CAD build for the part. Positions are in the model's coordinates, mm. A direction names the side the tool comes from. Coordinates: 2 decimals unless noted, no trailing zeros. Loops run counter-clockwise (first coordinate to the right, second up) from the corner with the lowest first, then second, coordinate; pieces in that order, holes last. Notation, with made-up numbers: (30, -39.5) -> (45, -39.5) arc R33 cw to (45, -7.5) -> close; hole circle Ø1 at (5.25, -13.75). An arc over 180 degrees is marked (long way). Answer as CSV lines item,"result". Start each with the question number.
```python
from build123d import *

# Parameters (mm, degrees)
F0_R     = 1.75
F1_DEPTH = 1.6
F2_DEPTH = 7.6
F3_DEPTH = 7.5
F4_START = 2.5
F4_DEPTH = 4


with BuildPart() as f1:
    # F0 (on Front) → F1 (new body)
    with BuildSketch(Plane.XZ):
        Polygon((19.785, -8), (19.785, 8), (13.385, 8), (13.385, 1.4), (0.585, 1.4), (0.585, 8), (-19.785, 8), (-19.785, -8), align=None)
        with BuildLine():
            ThreePointArc((-15.685, 4.5846688069), (-19.135, 5), (-15.685, 5.4153311931))
            Line((-15.685, 5.4153311931), (-15.685, 6.3))
            Line((-15.685, 6.3), (-8.285, 6.3))
            Line((-8.285, 6.3), (-8.285, -6.3))
            Line((-8.285, -6.3), (-15.685, -6.3))
            Line((-15.685, -6.3), (-15.685, -5.4153311931))
            ThreePointArc((-15.685, -5.4153311931), (-19.135, -5), (-15.685, -4.5846688069))
            Line((-15.685, -4.5846688069), (-15.685, 4.5846688069))
        make_face(mode=Mode.SUBTRACT)
        with Locations((-2.515, 5)):
            Circle(F0_R, mode=Mode.SUBTRACT)
        with Locations((16.485, 5)):
            Circle(F0_R, mode=Mode.SUBTRACT)
    extrude(amount=F1_DEPTH)

    # F0 (on Front) → F2 (join)
    with BuildSketch(Plane.XZ):
        Polygon((13.385, 1.4), (13.385, 8), (1.585, 8), (1.2352894992, 8), (0.585, 8), (0.585, 1.4), align=None)
    extrude(amount=F2_DEPTH)

    # F0 (on Front) → F3 (join)
    with BuildSketch(Plane.XZ):
        with BuildLine():
            ThreePointArc((-15.685, 5.4153311931), (-15.6475449646, 5.2091650066), (-15.635, 5))
            ThreePointArc((-15.635, 5), (-15.6475449646, 4.7908349934), (-15.685, 4.5846688069))
            Line((-15.685, 4.5846688069), (-15.685, -4.5846688069))
            ThreePointArc((-15.685, -4.5846688069), (-15.6475449646, -4.7908349934), (-15.635, -5))
            ThreePointArc((-15.635, -5), (-15.6475449646, -5.2091650066), (-15.685, -5.4153311931))
            Line((-15.685, -5.4153311931), (-15.685, -6.3))
            Line((-15.685, -6.3), (-8.285, -6.3))
            Line((-8.285, -6.3), (-8.285, 6.3))
            Line((-8.285, 6.3), (-15.685, 6.3))
            Line((-15.685, 6.3), (-15.685, 5.4153311931))
        make_face()
    extrude(amount=F3_DEPTH)

    # F0 (on Front) → F4 (join)
    with BuildSketch(Plane.XZ.offset(F4_START)):
        Polygon((1.2352894992, 8), (1.585, 8), (13.585, 13), (16.585, 13), (16.585, 13.1444329156), (13.5819284966, 13.1444329156), align=None)
    extrude(amount=F4_DEPTH)


solid = f1.part
```
Q1. Probe probe 1 along X at (y, z) = (-3.5, 1.75) (3 decimals); probe 2 along Y at (x, z) = (-13, -4); probe 3 along Z at (x, y) = (15, -0.25). List the from-to ranges inside material, lowest first. Write a range as from..to.
Q2. Saw through at C-C (x = 3). List the corners of the cut face in (y, z).
Q3. Two-plate mould, pull along Z, no slides. Class faces 1 (the flat face through (-12, -7.5, 0)), 2 (the cylindrical face through (-2.89, -0.79, 3.29)), 3 (the flat face through (0, -1, -8)): pulls with the +Z half, pulls with the -Z half, needs draft (parallel to the pull), parting line crosses it, or undercut.
Q4. Saw through at D-D (z = -1.75). List the corners of the cut face in (x, y) (3 decimals).
Q5. Which spindle directions (+Z, -Z, +X, -X, +Y, -Y) get a long thin tool onto all of the face, cutting with end or side? Do faces 4 (the flat face through (-15.685, -5, 6)), 5 (the flat face through (7, -7.6, 5)), 6 (the flat face through (13.385, -5, 5)), 7 (the flat face through (-12, -5, 6.3)), 8 (the flat face through (0.585, -5, 5)). Say none if no direction does.
Q6. Saw through at B-B (x = -13). List the corners of the cut face in (y, z), and give its area (3 significant figures).
Q7. Saw through at A-A (y = -3.25). List the corners of the cut face in (x, z) (3 decimals).
Q8. Pin check, flat tips, straight feed: pin 1 Ø3 at (x, y) = (-13.5, -5.5) entering from +Z; pin 2 Ø1.8 at (y, z) = (-5.5, -1.5) entering from +X (3 decimals); pin 3 Ø1.8 at (y, z) = (-4, -2) entering from -X (3 decimals); pin 4 Ø1.5 at (x, z) = (7, 2) entering from +Y. Stop position of each tip, or through.
Ans:
1,probe 1,"x = -15.685..-8.285, 0.585..13.385"
1,probe 2,"y = -7.5..0"
1,probe 3,"z = -8..4.07, 5.93..8"
2,outline,"(-7.6, 1.4) -> (-1.6, 1.4) -> (-1.6, -8) -> (0, -8) -> (0, 8) -> (-7.6, 8) -> close; (-6.5, 8.59) -> (-2.5, 8.59) -> (-2.5, 8.74) -> (-6.5, 8.74) -> close"
3,face 1,"needs draft"
3,face 2,"undercut"
3,face 3,"pulls with the -Z half"
4,outline,"(-19.785, -1.6) -> (-15.685, -1.6) -> (-15.685, -7.5) -> (-8.285, -7.5) -> (-8.285, -1.6) -> (19.785, -1.6) -> (19.785, 0) -> (-19.785, 0) -> close"
5,face 4,"+Z, -Z, -X, -Y"
5,face 5,"+Z, -Z, +X, -X, -Y"
5,face 6,"-Z, +X, -Y"
5,face 7,"+Z, -X, -Y"
5,face 8,"+Z, -Z, -Y"
6,outline,"(-7.5, -6.3) -> (-1.6, -6.3) -> (-1.6, -8) -> (0, -8) -> (0, 8) -> (-1.6, 8) -> (-1.6, 6.3) -> (-7.5, 6.3) -> close"
6,area,"99.9 mm²"
7,outline,"(-15.685, -6.3) -> (-8.285, -6.3) -> (-8.285, 6.3) -> (-15.685, 6.3) -> (-15.685, 5.415) arc R1.75 cw to (-15.685, 4.585) -> (-15.685, -4.585) arc R1.75 cw to (-15.685, -5.415) -> close; (0.585, 1.4) -> (13.385, 1.4) -> (13.385, 8) -> (1.585, 8) -> (13.585, 13) -> (16.585, 13) -> (16.585, 13.144) -> (13.582, 13.144) -> (1.235, 8) -> (0.585, 8) -> close"
8,pin 1,"stops at z = 6.3"
8,pin 2,"stops at x = -8.285"
8,pin 3,"stops at x = -15.685"
8,pin 4,"stops at y = 0"
